```python
from build123d import *

# Parameters (mm, degrees)
SKETCH1_W           = 95
SKETCH1_H           = 18
BOSS_EXTRUDE1_DEPTH = 5
SKETCH2_R           = 2
SKETCH2_W           = 95
SKETCH2_H           = 5
BOSS_EXTRUDE2_DEPTH = 2.5


with BuildPart() as part:
    # Sketch1 → Boss-Extrude1 (new body)
    with BuildSketch(Plane(origin=(0, 0, 0), x_dir=(1, 0, 0), z_dir=(0, 1, 0))):
        Rectangle(SKETCH1_W, SKETCH1_H)
        with BuildLine():
            Line((-38, 4), (-38, -4))
            ThreePointArc((-38, -4), (-40, -6), (-42, -4))
            Line((-42, -4), (-42, 4))
            ThreePointArc((-42, 4), (-40, 6), (-38, 4))
        make_face(mode=Mode.SUBTRACT)
        with BuildLine():
            Line((42, 4), (42, -4))
            ThreePointArc((42, -4), (40, -6), (38, -4))
            Line((38, -4), (38, 4))
            ThreePointArc((38, 4), (40, 6), (42, 4))
        make_face(mode=Mode.SUBTRACT)
    extrude(amount=BOSS_EXTRUDE1_DEPTH)

    # Sketch2 → Boss-Extrude2 (add)
    # profile 1 of 2: a face of its own
    with BuildSketch(Plane.XY.offset(9)):
        with BuildLine():
            Line((-52.5, -14.5), (-36.769552622, -14.5))
            ThreePointArc((-36.769552622, -14.5), (0, -1.5), (36.769552622, -14.5))
            Line((36.769552622, -14.5), (52.5, -14.5))
            ThreePointArc((52.5, -14.5), (57.449747468, -12.449747468), (59.5, -7.5))
            Line((59.5, -7.5), (59.5, 5))
            Line((59.5, 5), (47.5, 5))
            Line((47.5, 5), (47.5, 0))
            Line((47.5, 0), (-47.5, 0))
            Line((-47.5, 0), (-47.5, 5))
            Line((-47.5, 5), (-59.5, 5))
            Line((-59.5, 5), (-59.5, -7.5))
            ThreePointArc((-59.5, -7.5), (-57.449747468, -12.449747468), (-52.5, -14.5))
        make_face()
        with Locations((-52.5, -7.5)):
            Circle(SKETCH2_R, mode=Mode.SUBTRACT)
        with Locations((52.5, -7.5)):
            Circle(SKETCH2_R, mode=Mode.SUBTRACT)
    # profile 2 of 2: a face of its own
    with BuildSketch(Plane.XY.offset(9)):
        with Locations((0, 2.5)):
            Rectangle(SKETCH2_W, SKETCH2_H)
    extrude(amount=BOSS_EXTRUDE2_DEPTH)


solid = part.part
```
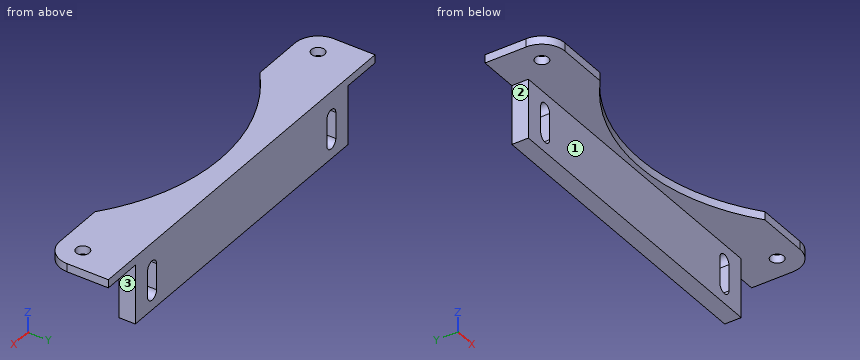
Design review of the part built by this model. Coordinates are the model's own, in mm. Face numbers are marked on the shaded views. Round coordinates to 2 decimals unless told otherwise and drop trailing zeros. Order: outer loops, then holes, each group sorted by start corner. A loop starts at its lowest first (then second) coordinate and runs counter-clockwise, first axis right, second up. Notation, with made-up numbers: (41.5, 27.5) - (66.5, 27.5) arc R18 cw to (66.5, 55.5) - close; hole circle Ø4 at (30, 60.5). An arc over 180 degrees is marked (long way). Return JSON: item names as keys, results as strings.
Q1. Wall thickness on L1, parallel to Y at x = -52.5, z = 10.05; L2, parallel to X at y = -6, z = 10.25; L3, parallel to Z at x = -49.5, y = -9: over which ranges is each line inside the solid? List them lowest first. Write a range as [from, to].
Computed values:
{"L1": "y = [-14.5, -9.5], [-5.5, 5]", "L2": "x = [-59.5, -53.82], [-51.18, -22.5], [22.5, 51.18], [53.82, 59.5]", "L3": "z = [9, 11.5]"}
Q2. The part is to be moulded in two halves that separate along X. For the marked faces 1, 2 and 3, say which applies: pulls with the +X half, pulls with the -X half, needs draft (parallel to the pull), parting line crosses it, or undercut.
Computed values:
{"face 1": "needs draft", "face 2": "pulls with the -X half", "face 3": "pulls with the +X half"}
Q3. Consider section C-C on x = 45. Write out the cut boundary in (y, z), plus the area to 3 significant figures.
Computed values:
{"outline": "(-14.5, 9) - (0, 9) - (0, -9) - (5, -9) - (5, 11.5) - (-14.5, 11.5) - close", "area": "139 mm2"}
Q4. For pin 1 Ø2.5 at (y, z) = (2, 0.5) entering from +X; pin 2 Ø1.5 at (y, z) = (2.5, 1.5) entering from -X; pin 3 Ø5 at (x, y) = (-52.5, -7.5) entering from -Z; pin 4 Ø8 at (x, z) = (41.5, 2.5) entering from +Y, all flat-tipped, find the tip position at first contact; note any pin that passes through.
Computed values:
{"pin 1": "stops at x = 47.5", "pin 2": "stops at x = -47.5", "pin 3": "stops at z = 9", "pin 4": "stops at y = 5"}
Q5. Consider section A-A on x = -40. Write out the cut boundary in (y, z), plus the area to 4 significant figures.
Computed values:
{"outline": "(-14.5, 9) - (0, 9) - (0, 6) - (5, 6) - (5, 11.5) - (-14.5, 11.5) - close; (0, -9) - (5, -9) - (5, -6) - (0, -6) - close", "area": "78.75 mm2"}
Q6. Consider section B-B on z = 5. Write out the cut boundary in (x, y).
Computed values:
{"outline": "(-47.5, 0) - (-41.73, 0) - (-41.73, 5) - (-47.5, 5) - close; (-38.27, 0) - (38.27, 0) - (38.27, 5) - (-38.27, 5) - close; (41.73, 0) - (47.5, 0) - (47.5, 5) - (41.73, 5) - close"}
Q7. Consider section D-D on x = 3. Write out the cut boundary in (y, z).
Computed values:
{"outline": "(-1.58, 9) - (0, 9) - (0, -9) - (5, -9) - (5, 11.5) - (-1.58, 11.5) - close"}
